from build123d import *

# Parameters (mm, degrees)
ESTRUSIONE_ESTRUSIONE1_DEPTH = 40
SCHIZZO2_R                   = 1.5
TAGLIO_ESTRUSIONE1_DEPTH     = 74.006848994
RACCORDO1_R                  = 3
RACCORDO2_R                  = 20
SCHIZZO3_R                   = 1.75
TAGLIO_ESTRUSIONE2_DEPTH     = 73.801098893
RACCORDO3_R                  = 3


with BuildPart() as part:
    # Schizzo1 → Estrusione-Estrusione1 (new body)
    with BuildSketch(Plane(origin=(0, 0, 0), x_dir=(1, 0, 0), z_dir=(0, 1, 0))):
        Polygon((0, 0), (0, 47), (3, 47), (3, 3), (42, 3), (42, 0), align=None)
    extrude(amount=ESTRUSIONE_ESTRUSIONE1_DEPTH)

    # Schizzo2 → Taglio-Estrusione1 (cut, through all)
    with BuildSketch(Plane(origin=(3, 0, 0), x_dir=(0, 0, -1), z_dir=(1, 0, 0))):
        with Locations((25, 4.5)):
            Circle(SCHIZZO2_R)
        with Locations((11.576606241, 12.25)):
            Circle(SCHIZZO2_R)
        with Locations((11.576606241, 27.75)):
            Circle(SCHIZZO2_R)
        with Locations((25, 35.5)):
            Circle(SCHIZZO2_R)
        with Locations((38.423393759, 27.75)):
            Circle(SCHIZZO2_R)
        with Locations((38.423393759, 12.25)):
            Circle(SCHIZZO2_R)
        with BuildLine():
            Line((18, 26.5), (32, 26.5))
            ThreePointArc((32, 26.5), (38.5, 20), (32, 13.5))
            Line((32, 13.5), (18, 13.5))
            ThreePointArc((18, 13.5), (11.5, 20), (18, 26.5))
        make_face()
    extrude(amount=-TAGLIO_ESTRUSIONE1_DEPTH, mode=Mode.SUBTRACT)

    # Raccordo1
    raccordo1_edges = [part.edges().sort_by_distance(p)[0] for p in [
        (0, 20, 0),
        (3, 20, -3),
    ]]
    fillet(raccordo1_edges, radius=RACCORDO1_R)

    # Raccordo2
    raccordo2_edges = [part.edges().sort_by_distance(p)[0] for p in [
        (1.5, 0, -47),
        (1.5, 40, -47),
    ]]
    fillet(raccordo2_edges, radius=RACCORDO2_R - 0.0001)  # a hair under: the kernel refuses the full size

    # Schizzo3 → Taglio-Estrusione2 (cut, through all)
    with BuildSketch(Plane(origin=(0, 0, -3), x_dir=(-1, 0, 0), z_dir=(0, 0, -1))):
        with Locations((-33.75, 34.95)):
            Circle(SCHIZZO3_R)
        with Locations((-9.75, 34.95)):
            Circle(SCHIZZO3_R)
        with Locations(Location((-9.75, 5.05, 0), (0, 0, 180))):
            Circle(SCHIZZO3_R)
        with Locations(Location((-33.75, 5.05, 0), (0, 0, 180))):
            Circle(SCHIZZO3_R)
    extrude(amount=-TAGLIO_ESTRUSIONE2_DEPTH, mode=Mode.SUBTRACT)

    # Raccordo3
    raccordo3_edges = [part.edges().sort_by_distance(p)[0] for p in [
        (42, 0, -1.5),
        (42, 40, -1.5),
    ]]
    fillet(raccordo3_edges, radius=RACCORDO3_R)


solid = part.part
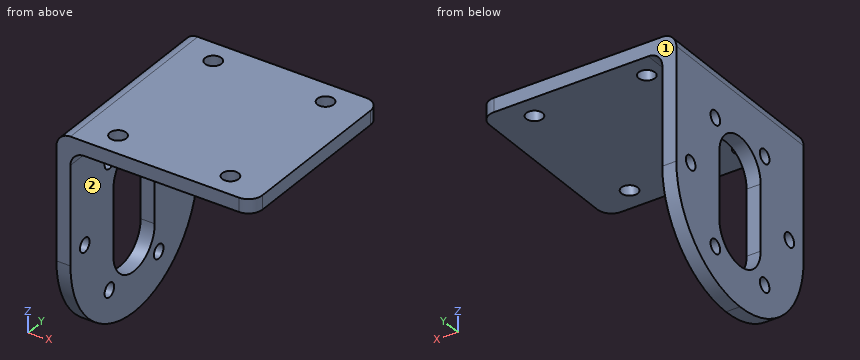
Check sheet for the modelled part. Datum: model origin and axes. Units: mm. Face numbers are marked on the shaded views. A direction names the side the tool comes from. Coordinates: 2 decimals unless noted, no trailing zeros. Loops run counter-clockwise (first coordinate to the right, second up) from the corner with the lowest first, then second, coordinate; pieces in that order, holes last. Notation, with made-up numbers: (30.25, 33) -> (67.25, 33) arc R28 cw to (67.25, 71) -> close; hole circle Ø3 at (75, 53.5). An arc over 180 degrees is marked (long way). Answer in a Markdown table with one row per item.
1. Sectioned sample at D-D, the plane y = 31. Record the boundary of the cut face in (x, z), then the cut area to 3 significant figures.
Check values:
| item | result |
|---|---|
| outline | (0, -43.7) -> (3, -43.7) -> (3, -6) arc R3 cw to (6, -3) -> (42, -3) -> (42, 0) -> (3, 0) arc R3 ccw to (0, -3) -> close |
| area | 248 mm2 |
2. Sectioned sample at C-C, the plane z = -31. Record the boundary of the cut face in (x, y), then the cut area to 3 significant figures.
Check values:
| item | result |
|---|---|
| outline | (0, 0.4) -> (3, 0.4) -> (3, 13.5) -> (0, 13.5) -> close; (0, 26.5) -> (3, 26.5) -> (3, 39.6) -> (0, 39.6) -> close |
| area | 78.6 mm2 |
3. Sectioned sample at B-B, the plane z = -25. Record the boundary of the cut face in (x, y).
Check values:
| item | result |
|---|---|
| outline | (0, 0) -> (3, 0) -> (3, 3) -> (0, 3) -> close; (0, 6) -> (3, 6) -> (3, 13.5) -> (0, 13.5) -> close; (0, 26.5) -> (3, 26.5) -> (3, 34) -> (0, 34) -> close; (0, 37) -> (3, 37) -> (3, 40) -> (0, 40) -> close |
4. Go/stop test with flat-tipped pins: pin 1 (2.5 mm diameter, centred on y = 12.25, z = -11.58, fed in from +X); pin 2 (12 mm diameter, centred on y = 5, z = -29.5, fed in from +X); pin 3 (12 mm diameter, centred on x = 22.5, y = 31, fed in from -Z). Record where each tip stops, or that it passes through.
Check values:
| item | result |
|---|---|
| pin 1 | passes through |
| pin 2 | stops at x = 3 |
| pin 3 | stops at z = -3 |
5. Access from +Z, -Z, +X, -X, +Y, -Y to the whole of each face (thin tool, end or side, straight path). Record for the marked faces 1 and 2.
Check values:
| item | result |
|---|---|
| face 1 | +Z, -Z, +X, -X, +Y |
| face 2 | -Z, +X, +Y, -Y |
6. Material ranges on line 1 along Y through (x, z) = (1.2, -25); line 2 along X through (y, z) = (5, -2); line 3 along Z through (x, y) = (7, 35), recorded low to high. Write a range as [from, to].
Check values:
| item | result |
|---|---|
| line 1 | y = [0, 3], [6, 13.5], [26.5, 34], [37, 40] |
| line 2 | x = [0.17, 8], [11.5, 32], [35.5, 42] |
| line 3 | z = [-3, 0] |
7. Sectioned sample at A-A, the plane x = 9.75. Record the boundary of the cut face in (y, z), then the cut area to 3 significant figures.
Check values:
| item | result |
|---|---|
| outline | (0, -3) -> (3.3, -3) -> (3.3, 0) -> (0, 0) -> close; (6.8, -3) -> (33.2, -3) -> (33.2, 0) -> (6.8, 0) -> close; (36.7, -3) -> (40, -3) -> (40, 0) -> (36.7, 0) -> close |
| area | 99.0 mm2 |
